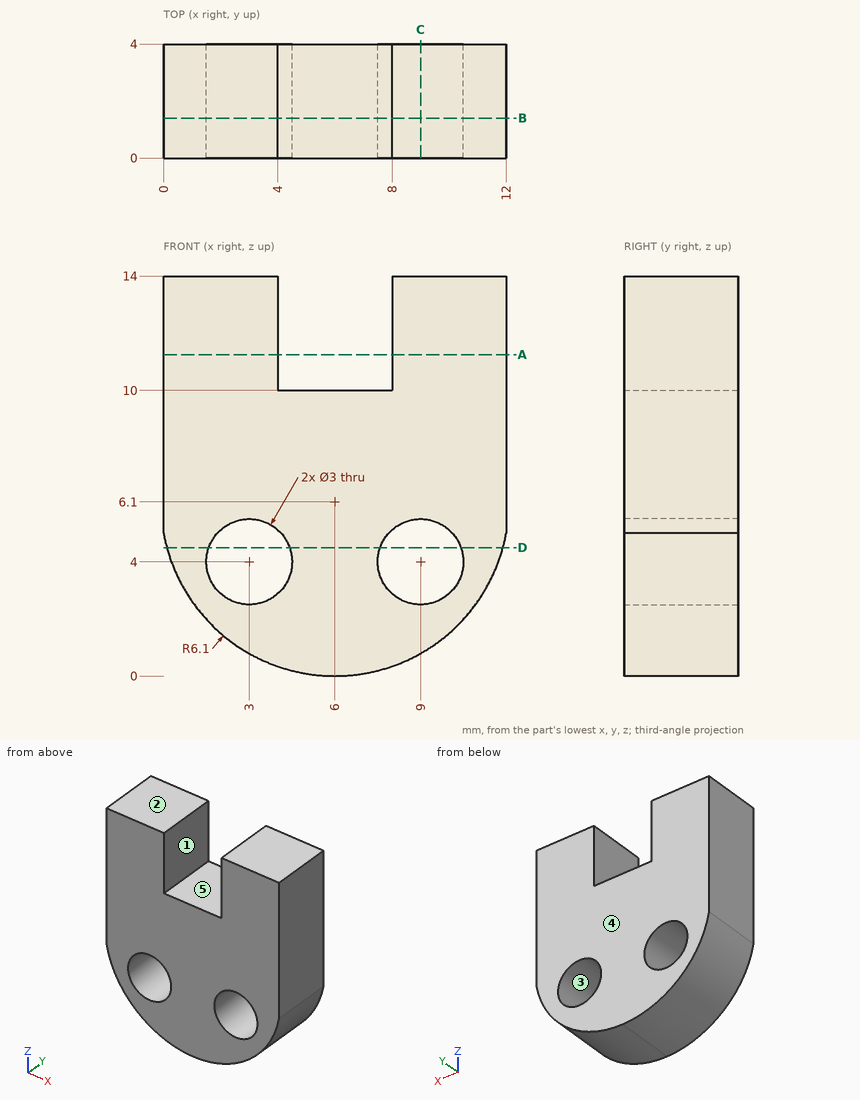
Study the drawing (mm; zero at the part's minimum x, y, z) and answer. A direction names the side the tool comes from. Give positions to 0.01 mm unless a question says otherwise; leave off trailing zeros. Write each loop counter-clockwise with the first axis right and the second up, starting at its lowest first coordinate (ties: lowest second). Pieces come first, ordered by that corner, then holes.
(1) A flat-ended cylindrical pin translates along its axis: pin 1 Ø2.5 at (x, z) = (3, 4) entering from -Y. Find the tip coordinate at first contact, or state that the pin passes through.
Final values:
pin 1: passes through
(2) The part is cut by section A-A on z = 11.25. Write down the section's boundary in (x, y), plus the area to 3 significant figures.
Final values:
outline: (0, 0) - (4, 0) - (4, 4) - (0, 4) - close; (8, 0) - (12, 0) - (12, 4) - (8, 4) - close
area: 32.0 mm2
(3) The part is cut by section D-D on z = 4.5. Write down the section's boundary in (x, y), plus the area to 3 significant figures.
Final values:
outline: (0.11, 0) - (1.59, 0) - (1.59, 4) - (0.11, 4) - close; (4.41, 0) - (7.59, 0) - (7.59, 4) - (4.41, 4) - close; (10.41, 0) - (11.89, 0) - (11.89, 4) - (10.41, 4) - close
area: 24.5 mm2
(4) Straight lines are drawn through the part: line 1 (X direction, y = 2.8, z = 4); line 2 (X direction, y = 1.5, z = 12.75); line 3 (X direction, y = 1.25, z = 3). For each, find the intervals that lie inside material, in ascending order.
Final values:
line 1: x = 0.27 to 1.5, 4.5 to 7.5, 10.5 to 11.73
line 2: x = 0 to 4, 8 to 12
line 3: x = 0.75 to 1.88, 4.12 to 7.88, 10.12 to 11.25
(5) The part is cut by section B-B on y = 1.4. Write down the section's boundary in (x, z).
Final values:
outline: (0, 5) arc R6.1 ccw to (12, 5) - (12, 14) - (8, 14) - (8, 10) - (4, 10) - (4, 14) - (0, 14) - close; hole circle Ø3 at (3, 4); hole circle Ø3 at (9, 4)
(6) Which of the six approach directions +Z, -Z, +X, -X, +Y, -Y give full straight-line access (tool end or side, diameter ignored) to the marked faces 4 and 5?
Final values:
face 4: +Z, -Z, +X, -X, +Y
face 5: +Z, +Y, -Y
(7) The mould has two halves that part along Z. Classify the marked faces 1, 2 and 3: pulls with the +Z half, pulls with the -Z half, needs draft (parallel to the pull), parting line crosses it, or undercut.
Final values:
face 1: needs draft
face 2: pulls with the +Z half
face 3: undercut
(8) The part is cut by section C-C on x = 9. Write down the section's boundary in (y, z), plus the area to 3 significant figures.
Final values:
outline: (0, 0.79) - (4, 0.79) - (4, 2.5) - (0, 2.5) - close; (0, 5.5) - (4, 5.5) - (4, 14) - (0, 14) - close
area: 40.8 mm2
